Geometry check sheet. Reference: the model listing, model coordinates, mm. Coordinates: 2 decimals unless noted, no trailing zeros. Loops run counter-clockwise (first coordinate to the right, second up) from the corner with the lowest first, then second, coordinate; pieces in that order, holes last.
from build123d import *

# Parameters (mm, degrees)
BOSS_EXTRUDE1_DEPTH = 72
BOSS_EXTRUDE2_DEPTH = 0.25
BOSS_EXTRUDE3_DEPTH = 0.25


with BuildPart() as part:
    # Sketch2 → Boss-Extrude1 (new, symmetric)
    with BuildSketch(Plane.XY):
        with BuildLine():
            Line((13.840423978, -6.020852528), (10.273266414, -0.926423564))
            ThreePointArc((10.273266414, -0.926423564), (9.915862983, -0.612989167), (9.45411437, -0.5))
            Line((9.45411437, -0.5), (-9.45411437, -0.5))
            ThreePointArc((-9.45411437, -0.5), (-9.915862983, -0.612989167), (-10.273266414, -0.926423564))
            Line((-10.273266414, -0.926423564), (-13.840423978, -6.020852528))
            Line((-13.840423978, -6.020852528), (-14.25, -5.73406431))
            Line((-14.25, -5.73406431), (-10.533549939, -0.426423564))
            ThreePointArc((-10.533549939, -0.426423564), (-10.176146508, -0.112989167), (-9.714397895, 0))
            Line((-9.714397895, 0), (9.714397895, 0))
            ThreePointArc((9.714397895, 0), (10.176146508, -0.112989167), (10.533549939, -0.426423564))
            Line((10.533549939, -0.426423564), (14.25, -5.73406431))
            Line((14.25, -5.73406431), (13.840423978, -6.020852528))
        make_face()
    extrude(amount=BOSS_EXTRUDE1_DEPTH, both=True)

    # Sketch3 → Boss-Extrude2 (add, symmetric)
    with BuildSketch(Plane(origin=(6.662976551, 4.665466408, 0), x_dir=(0, 0, -1), z_dir=(0.8191520442889926, 0.5735764363510449, 0))):
        with BuildLine():
            Line((-72, -6.651385295), (-75.5, -6.651385295))
            ThreePointArc((-75.5, -6.651385295), (-75.853553391, -6.797831905), (-76, -7.151385295))
            Line((-76, -7.151385295), (-76, -12.37053472))
            ThreePointArc((-76, -12.37053472), (-75.853553391, -12.72408811), (-75.5, -12.87053472))
            Line((-75.5, -12.87053472), (-72, -12.87053472))
            Line((-72, -12.87053472), (-72, -6.651385295))
        make_face()
        with BuildLine():
            Line((72, -12.87053472), (72, -6.651385295))
            Line((72, -6.651385295), (75.5, -6.651385295))
            ThreePointArc((75.5, -6.651385295), (75.853553391, -6.797831905), (76, -7.151385295))
            Line((76, -7.151385295), (76, -12.37053472))
            ThreePointArc((76, -12.37053472), (75.853553391, -12.72408811), (75.5, -12.87053472))
            Line((75.5, -12.87053472), (72, -12.87053472))
        make_face()
    extrude(amount=BOSS_EXTRUDE2_DEPTH, both=True)

    # Sketch4 → Boss-Extrude3 (add, symmetric)
    with BuildSketch(Plane(origin=(-6.662976551, 4.665466408, 0), x_dir=(0, 0, 1), z_dir=(-0.819152044288993, 0.5735764363510446, 0))):
        with BuildLine():
            Line((-72, -6.651385295), (-75.5, -6.651385295))
            ThreePointArc((-75.5, -6.651385295), (-75.853553391, -6.797831905), (-76, -7.151385295))
            Line((-76, -7.151385295), (-76, -12.37053472))
            ThreePointArc((-76, -12.37053472), (-75.853553391, -12.72408811), (-75.5, -12.87053472))
            Line((-75.5, -12.87053472), (-72, -12.87053472))
            Line((-72, -12.87053472), (-72, -6.651385295))
        make_face()
        with BuildLine():
            Line((72, -12.87053472), (72, -6.651385295))
            Line((72, -6.651385295), (75.5, -6.651385295))
            ThreePointArc((75.5, -6.651385295), (75.853553391, -6.797831905), (76, -7.151385295))
            Line((76, -7.151385295), (76, -12.37053472))
            ThreePointArc((76, -12.37053472), (75.853553391, -12.72408811), (75.5, -12.87053472))
            Line((75.5, -12.87053472), (72, -12.87053472))
        make_face()
    extrude(amount=BOSS_EXTRUDE3_DEPTH, both=True)


solid = part.part
(1) Gauge pin test, flat ends, axial feed: pin 1 Ø0.7 at (x, y) = (-1.5, -0.5) entering from -Z; pin 2 Ø2 at (y, z) = (-0.5, 56.5) entering from +X; pin 3 Ø3 at (x, y) = (-10.5, -4.5) entering from +Z; pin 4 Ø1.5 at (x, z) = (-3, 2.5) entering from -Y. Record the tip position at first contact, or that the pin passes through.
Findings:
pin 1: stops at z = -72
pin 2: stops at x = 11.29
pin 3: passes through
pin 4: stops at y = -0.5
(2) Scan lines: L1, parallel to Y at x = 0.75, z = 0; L2, parallel to X at y = -2.5, z = -26.5; L3, parallel to X at y = -2, z = -51 (3 decimals). Record each from-to range of solid material in increasing order.
Findings:
L1: y = -0.5 to 0
L2: x = -11.99 to -11.38, 11.38 to 11.99
L3: x = -11.635 to -11.025, 11.025 to 11.635
(3) Sectioned sample at C-C on x = 6.5. Record the cut outline in (y, z), and give its area (3 significant figures).
Findings:
outline: (-0.5, -72) - (0, -72) - (0, 72) - (-0.5, 72) - close
area: 72.0 mm2
(4) Sectioned sample at A-A on z = -45. Record the cut outline in (x, y).
Findings:
outline: (-14.25, -5.73) - (-13.84, -6.02) - (-10.27, -0.93) arc R1 cw to (-9.45, -0.5) - (9.45, -0.5) arc R1 cw to (10.27, -0.93) - (13.84, -6.02) - (14.25, -5.73) - (10.53, -0.43) arc R1 ccw to (9.71, 0) - (-9.71, 0) arc R1 ccw to (-10.53, -0.43) - close
(5) Draft check along X on faces 1 (the flat face through (12, -3, 76)), 2 (the flat face through (0, -0.5, 1)). Enter one of: +X half, -X half, draft (parallel to the pull), parting line (faces both ways), or undercut.
Findings:
face 1: draft
face 2: undercut
(6) Sectioned sample at B-B on y = -4. Record the cut outline in (x, z), and give its area (3 significant figures).
Findings:
outline: (-13.04, -76) - (-12.43, -76) - (-12.43, 76) - (-13.04, 76) - close; (12.43, -76) - (13.04, -76) - (13.04, 76) - (12.43, 76) - close
area: 186 mm2
